Geometry: final body of the model. Coordinates: model frame, mm. Give positions to 0.01 mm unless a question says otherwise; leave off trailing zeros. Write each loop counter-clockwise with the first axis right and the second up, starting at its lowest first coordinate (ties: lowest second). Pieces come first, ordered by that corner, then holes.
Q1. Cut plane B-B on y = 1.65. Return the cut outline in (x, z), plus the area to 3 significant figures.
Q2. Cut plane A-A on z = 0. Return the cut outline in (x, y) (3 decimals).
Q3. Line query: L1, parallel to X at y = 2.25, z = -1; L2, parallel to Z at x = -1, y = 1.8. Output: solid intervals per line, ascending.
Q4. Cut plane C-C on x = -110.5. Return the cut outline in (y, z) (3 decimals), plus the area to 3 significant figures.
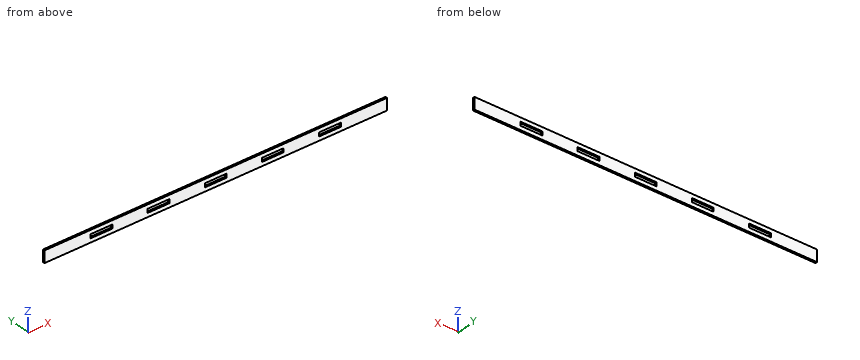
```python
from build123d import *

# Parameters (mm, degrees)
SKETCH1_W           = 596.9
SKETCH1_H           = 20.828
BOSS_EXTRUDE1_DEPTH = 3.175
SKETCH5_W           = 38.1
SKETCH5_H           = 6.858
CUT_EXTRUDE2_DEPTH  = 299.648513341


with BuildPart() as part:
    # Sketch1 → Boss-Extrude1 (new body)
    with BuildSketch(Plane(origin=(0, 0, 0), x_dir=(1, 0, 0), z_dir=(0, 1, 0))):
        Rectangle(SKETCH1_W, SKETCH1_H)
    extrude(amount=BOSS_EXTRUDE1_DEPTH)

    # Sketch5 → Cut-Extrude2 (cut, through all)
    with BuildSketch(Plane(origin=(0, 3.175, 0), x_dir=(1, 0, 0), z_dir=(0, 1, 0))):
        with Locations((-198.966666582, 0)):
            Rectangle(SKETCH5_W, SKETCH5_H)
        with Locations((-99.483333164, 0)):
            Rectangle(SKETCH5_W, SKETCH5_H)
        with Locations((1.69e-07, 0)):
            Rectangle(SKETCH5_W, SKETCH5_H)
        with Locations((99.483333333, 0)):
            Rectangle(SKETCH5_W, SKETCH5_H)
        with Locations((198.966666667, 0)):
            Rectangle(SKETCH5_W, SKETCH5_H)
    extrude(amount=-CUT_EXTRUDE2_DEPTH, mode=Mode.SUBTRACT)


solid = part.part
```
Data:
1. outline: (-298.45, -10.41) - (298.45, -10.41) - (298.45, 10.41) - (-298.45, 10.41) - close; hole (-218.02, -3.43) - (-179.92, -3.43) - (-179.92, 3.43) - (-218.02, 3.43) - close; hole (-118.53, -3.43) - (-80.43, -3.43) - (-80.43, 3.43) - (-118.53, 3.43) - close; hole (-19.05, -3.43) - (19.05, -3.43) - (19.05, 3.43) - (-19.05, 3.43) - close; hole (80.43, -3.43) - (118.53, -3.43) - (118.53, 3.43) - (80.43, 3.43) - close; hole (179.92, -3.43) - (218.02, -3.43) - (218.02, 3.43) - (179.92, 3.43) - close
1. area: 11,100 mm2
2. outline: (-298.45, 0) - (-218.017, 0) - (-218.017, 3.175) - (-298.45, 3.175) - close; (-179.917, 0) - (-118.533, 0) - (-118.533, 3.175) - (-179.917, 3.175) - close; (-80.433, 0) - (-19.05, 0) - (-19.05, 3.175) - (-80.433, 3.175) - close; (19.05, 0) - (80.433, 0) - (80.433, 3.175) - (19.05, 3.175) - close; (118.533, 0) - (179.917, 0) - (179.917, 3.175) - (118.533, 3.175) - close; (218.017, 0) - (298.45, 0) - (298.45, 3.175) - (218.017, 3.175) - close
3. L1: x = -298.45 to -218.02, -179.92 to -118.53, -80.43 to -19.05, 19.05 to 80.43, 118.53 to 179.92, 218.02 to 298.45
3. L2: z = -10.41 to -3.43, 3.43 to 10.41
4. outline: (0, -10.414) - (3.175, -10.414) - (3.175, -3.429) - (0, -3.429) - close; (0, 3.429) - (3.175, 3.429) - (3.175, 10.414) - (0, 10.414) - close
4. area: 44.4 mm2
